from build123d import *

# Parameters (mm, degrees)
BOSS_EXTRUDE1_DEPTH     = 20
FILLET1_R               = 4
SKETCH2_R               = 2.75
CUT_EXTRUDE1_DEPTH      = 1.5
LPATTERN1_COUNT         = 2
LPATTERN1_PITCH         = 30
CUT_EXTRUDE2_DEPTH      = 35.369317712
CUT_EXTRUDE2_DEPTH_BACK = 35.369317712
WRAP1_DEPTH             = 1


# Read off the part's stored shape, not the designer's step: Wrap1
with BuildPart() as part:
    # Sketch1 → Boss-Extrude1 (new body)
    with BuildSketch(Plane(origin=(0, 0, 0), x_dir=(1, 0, 0), z_dir=(0, 1, 0))):
        with BuildLine():
            Line((22.5, -5), (-22.5, -5))
            ThreePointArc((-22.5, -5), (-27.5, 0), (-22.5, 5))
            Line((-22.5, 5), (22.5, 5))
            ThreePointArc((22.5, 5), (27.5, 0), (22.5, -5))
        make_face()
    extrude(amount=BOSS_EXTRUDE1_DEPTH)

    # Fillet1
    fillet1_edges = [part.edges().sort_by_distance(p)[0] for p in [
        (-27.5, 20, 0),
        (0, 20, 5),
        (27.5, 20, 0),
        (0, 20, -5),
    ]]
    fillet(fillet1_edges, radius=FILLET1_R)

    # Sketch2 → Cut-Extrude1 (cut)
    with BuildSketch(Plane.XZ):
        with Locations(Location((-22.5, 0, 0), (0, 0, 270))):
            Circle(SKETCH2_R)
    cut_extrude1 = extrude(amount=-CUT_EXTRUDE1_DEPTH, mode=Mode.SUBTRACT)

    # LPattern1: Cut-Extrude1 ×2
    with Locations(*[(i * LPATTERN1_PITCH, 0, 0) for i in range(1, LPATTERN1_COUNT)]):
        add(cut_extrude1, mode=Mode.SUBTRACT)

    # Sketch3 → Cut-Extrude2 (cut, two sides: drawn at the far end of the back side and taken through both)
    with BuildSketch(Plane.XY.offset(-CUT_EXTRUDE2_DEPTH_BACK)):
        with BuildLine():
            Line((-5, 23), (5, 23))
            ThreePointArc((5, 23), (8, 20), (5, 17))
            Line((5, 17), (-5, 17))
            ThreePointArc((-5, 17), (-8, 20), (-5, 23))
        make_face()
    extrude(amount=CUT_EXTRUDE2_DEPTH + CUT_EXTRUDE2_DEPTH_BACK, mode=Mode.SUBTRACT)

    # Wrap1 outline → Wrap1 (add)
    with BuildSketch(Plane(origin=(0, 17, 0), x_dir=(1, 0, 0), z_dir=(0, 1, 0))):
        with BuildLine():
            add(Edge.make_bspline(
                [(0.968558604, -2.112404227), (1.023340463, -2.110381468), (1.128135866, -2.106512015), (1.275421614, -2.065066433), (1.40411806, -1.999153831), (1.494113345, -1.918796765), (1.555259283, -1.8377784), (1.600182088, -1.761379971), (1.643056037, -1.669468115), (1.68410688, -1.562162987), (1.724115658, -1.439672484), (1.762787282, -1.301883834), (1.796828359, -1.147944523), (1.819117415, -1.040313742), (1.830738091, -0.984199098)],
                knots=[0, 0, 0, 0, 0.10403341, 0.199011557, 0.288612319, 0.377191825, 0.425797175, 0.481425289, 0.545557079, 0.61863331, 0.699984683, 0.790771883, 0.890916323, 1, 1, 1, 1], degree=3))
            Line((0.968558604, -2.112404227), (-1.502595242, -2.112404227))
            add(Edge.make_bspline(
                [(0.359584245, -0.57875038), (0.287589412, -0.631266446), (0.149119993, -0.732271876), (-0.052040125, -0.874957595), (-0.232151558, -1.010570949), (-0.396984875, -1.13231455), (-0.543079134, -1.243803459), (-0.672030163, -1.343433338), (-0.782764208, -1.43141572), (-0.961872458, -1.579798827), (-1.207220157, -1.798528227), (-1.40469562, -2.00837263), (-1.502595242, -2.112404227)],
                knots=[0, 0, 0, 0, 0.110593572, 0.212707314, 0.306051588, 0.390379305, 0.467018215, 0.534117187, 0.592614819, 0.642525788, 0.822780058, 1, 1, 1, 1], degree=3))
            add(Edge.make_bspline(
                [(2.103173989, 1.329903466), (2.066781163, 1.246346618), (1.99482956, 1.081147874), (1.86047631, 0.847661593), (1.71297016, 0.626020413), (1.571074283, 0.452909604), (1.445054335, 0.315568643), (1.334068385, 0.207346612), (1.208958187, 0.091994137), (1.069166496, -0.030104), (0.913592831, -0.158279882), (0.741560734, -0.29208501), (0.556771712, -0.435146764), (0.42660857, -0.529939289), (0.359584245, -0.57875038)],
                knots=[0, 0, 0, 0, 0.10413489, 0.205883221, 0.307528832, 0.408265615, 0.461433854, 0.520606469, 0.585444086, 0.656004792, 0.732803839, 0.815893726, 0.905198979, 1, 1, 1, 1], degree=3))
            add(Edge.make_bspline(
                [(2.258622707, 2.155223979), (2.256854974, 2.081406691), (2.253395008, 1.936924834), (2.223825952, 1.724789841), (2.174767432, 1.522306219), (2.126875674, 1.393600214), (2.103173989, 1.329903466)],
                knots=[0, 0, 0, 0, 0.261979501, 0.512769921, 0.758869279, 1, 1, 1, 1], degree=3))
            add(Edge.make_bspline(
                [(-0.061890114, 4.14400603), (0.022564629, 4.141920306), (0.18812583, 4.13783155), (0.430620451, 4.112847977), (0.660471364, 4.067558501), (0.878305178, 4.005888588), (1.082018473, 3.923000729), (1.274759097, 3.825795699), (1.453280397, 3.707304776), (1.618929442, 3.573545968), (1.768923738, 3.427244365), (1.900049838, 3.270535022), (2.011299511, 3.105351175), (2.101257211, 2.93081783), (2.172841542, 2.749020464), (2.221753805, 2.558426678), (2.253872753, 2.359840276), (2.257020026, 2.224263519), (2.258622707, 2.155223979)],
                knots=[0, 0, 0, 0, 0.074102612, 0.14526736, 0.21355926, 0.279416432, 0.343556942, 0.406228654, 0.468492489, 0.531146675, 0.592790073, 0.652016559, 0.710119813, 0.767135501, 0.823967905, 0.881147087, 0.939476717, 1, 1, 1, 1], degree=3))
            add(Edge.make_bspline(
                [(-1.906441396, 3.445288081), (-1.848306189, 3.501112989), (-1.732554849, 3.612264359), (-1.538609793, 3.754854821), (-1.330466242, 3.876473687), (-1.105791254, 3.973994027), (-0.866480346, 4.051164268), (-0.611446439, 4.105367467), (-0.341562002, 4.137488539), (-0.156530269, 4.14180053), (-0.061890114, 4.14400603)],
                knots=[0, 0, 0, 0, 0.119107626, 0.23715177, 0.355050392, 0.47498588, 0.598670295, 0.726365388, 0.860041186, 1, 1, 1, 1], degree=3))
            add(Edge.make_bspline(
                [(-2.459326011, 2.031826543), (-2.458122329, 2.10083777), (-2.455751672, 2.236755643), (-2.42704922, 2.435648535), (-2.383831572, 2.625974396), (-2.325084873, 2.808678323), (-2.245799792, 2.981581962), (-2.150493697, 3.146407777), (-2.038697096, 3.303051555), (-1.950794522, 3.397587797), (-1.906441396, 3.445288081)],
                knots=[0, 0, 0, 0, 0.132803649, 0.26155729, 0.386082589, 0.508400008, 0.630401232, 0.751619273, 0.874674186, 1, 1, 1, 1], degree=3))
            add(Edge.make_bspline(
                [(-1.520223447, 0.759390645), (-1.585420599, 0.763118791), (-1.713143024, 0.770422298), (-1.895082142, 0.836934937), (-2.058691576, 0.943915448), (-2.201841078, 1.092044894), (-2.320121913, 1.277705611), (-2.399559254, 1.501224402), (-2.452612405, 1.75530448), (-2.457009968, 1.936432658), (-2.459326011, 2.031826543)],
                knots=[0, 0, 0, 0, 0.110139331, 0.215764983, 0.323707128, 0.438906263, 0.562183724, 0.693638164, 0.838649921, 1, 1, 1, 1], degree=3))
            add(Edge.make_bspline(
                [(-0.613172165, 1.631185517), (-0.616054345, 1.570486701), (-0.621662157, 1.45238594), (-0.671323685, 1.283175242), (-0.754629801, 1.131365188), (-0.869218028, 1.000302814), (-1.00648217, 0.893380798), (-1.162575656, 0.81342959), (-1.336719307, 0.768952542), (-1.458017598, 0.762632021), (-1.520223447, 0.759390645)],
                knots=[0, 0, 0, 0, 0.129242333, 0.251464839, 0.372304265, 0.495878621, 0.620081591, 0.741344555, 0.867352775, 1, 1, 1, 1], degree=3))
            add(Edge.make_bspline(
                [(-1.273428575, 2.371570132), (-1.221111857, 2.356431424), (-1.121681232, 2.327659528), (-0.986315759, 2.264054818), (-0.872118751, 2.188748181), (-0.775565412, 2.103031066), (-0.702763657, 2.001965174), (-0.650977929, 1.888692008), (-0.61737495, 1.763975364), (-0.614599413, 1.676280399), (-0.613172165, 1.631185517)],
                knots=[0, 0, 0, 0, 0.151156851, 0.287281401, 0.413669873, 0.530293514, 0.644009236, 0.756908248, 0.874996313, 1, 1, 1, 1], degree=3))
            add(Edge.make_bspline(
                [(-1.659646524, 2.52701885), (-1.641908981, 2.5134804), (-1.599762076, 2.48131113), (-1.513799429, 2.446453071), (-1.403911325, 2.405291879), (-1.319666952, 2.383519902), (-1.273428575, 2.371570132)],
                knots=[0, 0, 0, 0, 0.159109439, 0.378066483, 0.65864549, 1, 1, 1, 1], degree=3))
            add(Edge.make_bspline(
                [(-1.741377293, 2.725736799), (-1.740702967, 2.705828636), (-1.739402264, 2.667427893), (-1.722346439, 2.613602242), (-1.696843256, 2.565494988), (-1.672067897, 2.539867464), (-1.659646524, 2.52701885)],
                knots=[0, 0, 0, 0, 0.268945253, 0.518766978, 0.758729042, 1, 1, 1, 1], degree=3))
            add(Edge.make_bspline(
                [(-0.509005498, 3.631185517), (-0.593702292, 3.627478268), (-0.757485819, 3.620309328), (-0.992510379, 3.565399378), (-1.204920463, 3.4708981), (-1.388970755, 3.342097951), (-1.54050767, 3.195942921), (-1.655393233, 3.044422755), (-1.727025811, 2.886507887), (-1.736695124, 2.778188345), (-1.741377293, 2.725736799)],
                knots=[0, 0, 0, 0, 0.151816317, 0.293576777, 0.429964406, 0.566304914, 0.694365033, 0.806085808, 0.906100976, 1, 1, 1, 1], degree=3))
            add(Edge.make_bspline(
                [(0.617597066, 2.220929107), (0.616798314, 2.277062503), (0.615251229, 2.385786079), (0.599863671, 2.542997259), (0.579004071, 2.690242583), (0.544058374, 2.826348498), (0.504153512, 2.954009696), (0.449772713, 3.069509609), (0.389899195, 3.176431124), (0.318093883, 3.271087373), (0.240513737, 3.356936451), (0.152380296, 3.428872442), (0.059506725, 3.491963217), (-0.040243661, 3.543993611), (-0.147906764, 3.581901434), (-0.261368703, 3.611540097), (-0.38306343, 3.626855058), (-0.466235221, 3.629714881), (-0.509005498, 3.631185517)],
                knots=[0, 0, 0, 0, 0.082284271, 0.159374645, 0.231497254, 0.300083139, 0.36523236, 0.427274673, 0.486932074, 0.544586116, 0.60112786, 0.656190593, 0.710940404, 0.765594865, 0.820607428, 0.877984079, 0.93725451, 1, 1, 1, 1], degree=3))
            add(Edge.make_bspline(
                [(0.205738091, 0.635993209), (0.238640814, 0.700768661), (0.303861654, 0.829168655), (0.385865127, 1.026897746), (0.459663901, 1.22391557), (0.516579645, 1.422967903), (0.561905142, 1.621957205), (0.593823909, 1.82108009), (0.613938148, 2.020726724), (0.616375849, 2.154108657), (0.617597066, 2.220929107)],
                knots=[0, 0, 0, 0, 0.131745637, 0.261150462, 0.388067803, 0.513189353, 0.636374668, 0.758087597, 0.878808958, 1, 1, 1, 1], degree=3))
            add(Edge.make_bspline(
                [(-1.116377293, -1.107596534), (-1.03496234, -1.013767374), (-0.878016077, -0.832889839), (-0.655626445, -0.569536189), (-0.456135085, -0.32390871), (-0.280159151, -0.096566641), (-0.125247461, 0.111659158), (0.00577288, 0.302221735), (0.116680709, 0.473318508), (0.177475044, 0.584367138), (0.205738091, 0.635993209)],
                knots=[0, 0, 0, 0, 0.170005554, 0.327725258, 0.471696803, 0.603008639, 0.721148947, 0.826797124, 0.919478664, 1, 1, 1, 1], degree=3))
            add(Edge.make_bspline(
                [(-2.664454216, -3.057917047), (-2.628698989, -3.000910883), (-2.55158858, -2.877970296), (-2.41479269, -2.688825323), (-2.259314405, -2.474715573), (-2.074551732, -2.243606397), (-1.870318919, -1.988170585), (-1.640593125, -1.712928149), (-1.387471618, -1.416348269), (-1.20904993, -1.213142224), (-1.116377293, -1.107596534)],
                knots=[0, 0, 0, 0, 0.080973991, 0.174630064, 0.280853316, 0.39944862, 0.530692677, 0.674513651, 0.830941638, 1, 1, 1, 1], degree=3))
            Line((-2.664454216, -3.057917047), (-2.664454216, -3.548301662))
            Line((-2.664454216, -3.548301662), (2.156058604, -3.548301662))
            Line((2.156058604, -3.548301662), (2.361186809, -0.984199098))
            Line((2.361186809, -0.984199098), (1.830738091, -0.984199098))
        make_face()
    extrude(amount=WRAP1_DEPTH)


solid = part.part
The model under review builds one solid part; all positions refer to its coordinate system, in mm. A direction names the side the tool comes from. Give positions to 0.01 mm unless a question says otherwise; leave off trailing zeros. Write each loop counter-clockwise with the first axis right and the second up, starting at its lowest first coordinate (ties: lowest second). Pieces come first, ordered by that corner, then holes.
1. Add section A-A, the plane x = -15. Write out the cut boundary in (y, z).
2. Add section D-D, the plane x = -7. Write out the cut boundary in (y, z).
3. Wall thickness on L1, parallel to X at y = 1.05, z = 0; L2, parallel to Y at x = 1, z = 1.75; L3, parallel to Y at x = -22.5, z = 0.5: over which ranges is each line inside the solid? List them lowest first.
4. Draft analysis for pull direction Z (two halves, no side actions). For faces 1 (the flat face through (-0.3, 17.5, 3.548)), 2 (the cylindrical face through (0.32, 16.3, -4.99)), 3 (the cylindrical face through (-7.1, 17.86, -0.07)), 4 (the flat face through (-0.2, 17.5, 2.112)), state which applies: +Z half, -Z half, draft (parallel to the pull), parting line (faces both ways), or undercut.
5. Tool access review of faces 5 (the flat face through (2.257, 17.493, 2.284)), 6 (the flat face through (-16, 20, 0)), 7 (the cylindrical face through (7.14, 17.9, -0.07)), 8 (the cylindrical face through (4.815, 0.74, 0.596)): name each direction out of +Z, -Z, +X, -X, +Y, -Y from which nothing blocks a thin tool from reaching the whole face with its end or side.
6. Add section B-B, the plane y = 2. Write out the cut boundary in (x, z).
7. For P1, Ø6, axis at y = 10.5, z = -3.5, coming from the +X side; P2, Ø4.5, axis at x = -22.5, z = 0, coming from the -Y side; P3, Ø0.8, axis at x = -0.5, y = 17.5, coming from the +Z side, all flat-tipped, find the tip position at first contact; note any pin that passes through.
8. Add section C-C, the plane x = 9. Write out the cut boundary in (y, z).
Worked answers:
1. outline: (0, -5) - (16, -5) arc R4 ccw to (20, -1) - (20, 1) arc R4 ccw to (16, 5) - (0, 5) - close
2. outline: (0, -5) - (16, -5) arc R4 ccw to (17.76, -4.59) - (17.76, 4.59) arc R4 ccw to (16, 5) - (0, 5) - close
3. L1: x = -27.5 to -25.25, -19.75 to 4.75, 10.25 to 27.5
3. L2: y = 0 to 17
3. L3: y = 1.5 to 20
4. face 1: +Z half
4. face 2: -Z half
4. face 3: draft
4. face 4: undercut
5. face 5: +Z, +Y
5. face 6: +Z, -Z, +X, -X, +Y
5. face 7: +Z, -Z, +Y
5. face 8: -Y
6. outline: (-22.5, -5) - (22.5, -5) arc R5 ccw to (22.5, 5) - (-22.5, 5) arc R5 ccw to start
7. P1: stops at x = 27.47
7. P2: stops at y = 1.5
7. P3: stops at z = 3.55
8. outline: (0, -5) - (16, -5) arc R4 ccw to (20, -1) - (20, 1) arc R4 ccw to (16, 5) - (0, 5) - (0, 2.3) - (1.5, 2.3) - (1.5, -2.3) - (0, -2.3) - close
